```python
from build123d import *

# Parameters (mm, degrees)
SKETCH1_W                    = 152.4
SKETCH1_H                    = 50.8
BOSS_EXTRUDE2_DEPTH          = 152.4
SHELL1_T                     = -12.7
SKETCH2_R                    = 3.877794573
BOSS_EXTRUDE3_DEPTH          = 6
M2_5X0_45_TAPPED_HOLE3_D     = 2.05
M2_5X0_45_TAPPED_HOLE3_DEPTH = 4.99999
M2_5X0_45_TAPPED_HOLE3_TIP   = 0.615882135


with BuildPart() as part:
    # Sketch1 → Boss-Extrude2 (new body)
    with BuildSketch(Plane.XY):
        with Locations((65.122807232, 229.754701441)):
            Rectangle(SKETCH1_W, SKETCH1_H)
    extrude(amount=BOSS_EXTRUDE2_DEPTH)

    # Shell1
    shell1_openings = [part.faces().sort_by_distance(p)[0] for p in [
        (65.122807232, 255.154701441, 76.2),
    ]]
    offset(amount=SHELL1_T, openings=shell1_openings, kind=Kind.INTERSECTION)

    # Sketch2 → Boss-Extrude3 (add)
    with BuildSketch(Plane(origin=(0, 217.054701441, 0), x_dir=(1, 0, 0), z_dir=(0, 1, 0))):
        with Locations(Location((32.002807193, -55.2, 0), (0, 0, 270))):
            Circle(SKETCH2_R)
        with BuildLine():
            Line((99.91232539, -51.7), (96.573289151, -51.7))
            ThreePointArc((96.573289151, -51.7), (95.500792432, -57.942014839), (101.742807271, -56.869518119))
            Line((101.742807271, -56.869518119), (101.742807271, -53.530481881))
            ThreePointArc((101.742807271, -53.530481881), (100.984822109, -52.457985161), (99.91232539, -51.7))
        make_face()
        with BuildLine():
            ThreePointArc((33.672325312, -100.7), (34.744822031, -94.457985161), (28.502807193, -95.530481881))
            Line((28.502807193, -95.530481881), (28.502807193, -98.869518119))
            ThreePointArc((28.502807193, -98.869518119), (29.260792354, -99.942014839), (30.333289073, -100.7))
            Line((30.333289073, -100.7), (33.672325312, -100.7))
        make_face()
        with BuildLine():
            Line((101.742807271, -98.869518119), (101.742807271, -95.530481881))
            ThreePointArc((101.742807271, -95.530481881), (95.500792432, -94.457985161), (96.573289151, -100.7))
            Line((96.573289151, -100.7), (99.91232539, -100.7))
            ThreePointArc((99.91232539, -100.7), (100.984822109, -99.942014839), (101.742807271, -98.869518119))
        make_face()
    extrude(amount=BOSS_EXTRUDE3_DEPTH)

    # M2.5x0.45 Tapped Hole3
    with Locations(Plane(origin=(0, 223.054701441, 0), x_dir=(1, 0, 0), z_dir=(0, 1, 0))):
        with Locations((32.002807193, -55.2), (98.242807271, -55.2), (98.242807271, -97.2), (32.002807193, -97.2)):
            Hole(M2_5X0_45_TAPPED_HOLE3_D / 2, depth=M2_5X0_45_TAPPED_HOLE3_DEPTH)
            with Locations((0, 0, -(M2_5X0_45_TAPPED_HOLE3_DEPTH + M2_5X0_45_TAPPED_HOLE3_TIP / 2))):  # 118° drill point
                Cone(0, M2_5X0_45_TAPPED_HOLE3_D / 2, M2_5X0_45_TAPPED_HOLE3_TIP, mode=Mode.SUBTRACT)


solid = part.part
```
Source: CAD feature listing. Evaluate the final solid. Frame: model axes, mm. A direction names the side the tool comes from. Round coordinates to 2 decimals unless told otherwise and drop trailing zeros. Loops run counter-clockwise (first coordinate to the right, second up) from the corner with the lowest first, then second, coordinate; pieces in that order, holes last. Notation, with made-up numbers: M -30,50 L 21,50 A22 ccw 21,74 Z; hole C 23,34 d10. An arc over 180 degrees is marked long. Use a Markdown table: item, result. Add a question column.
1. Contact query for flat-ended pins moving along their axis: P1, Ø8, axis at x = 30.5, z = 95.5, coming from the +Y side; P2, Ø3, axis at x = 76.5, z = 115.5, coming from the +Y side. Output: stop coordinate, or through.
2. Section query A-A on y = 221. Give the number of separate pieces and of enclosed holes in the cut face, then the cut area to 3 significant figures.
3. Section query C-C on y = 242.5. Return the cut outline in (x, z), then the cut area to 3 significant figures.
4. Line query: line 1 (X direction, y = 220.1, z = 55.2); line 2 (X direction, y = 219, z = 55); line 3 (Z direction, x = 116.5, y = 249). Output: solid intervals per line, ascending.
5. Reachability of faces 1 (the flat face through (64, 204.355, 75)), 2 (the flat face through (97, 223.055, 55)) from +Z, -Z, +X, -X, +Y, -Y: full face, straight path, thin tool, end or side. Return the list, or none.
6. Mould query, pull axis X, two halves, no side actions, for faces 3 (the flat face through (141.323, 229, 75)), 4 (the flat face through (64, 230, 152.4)), 5 (the cylindrical face through (95.43, 220.01, 57.87)), 6 (the cylindrical face through (34.817, 220.013, 94.532)). Classes: pulls with the +X half, pulls with the -X half, needs draft (parallel to the pull), parting line crosses it, or undercut.
7. Section query D-D on z = 38.5. Return the cut outline in (x, y).
8. Section query B-B on x = 23. Return the cut outline in (y, z), then the cut area to 3 significant figures.
Reported:
| question | item | result |
|---|---|---|
| 1 | P1 | stops at y = 223.05 |
| 1 | P2 | stops at y = 217.05 |
| 2 | separate pieces | 5 |
| 2 | enclosed holes | 5 |
| 2 | area | 7,270 mm² |
| 3 | outline | M -11.08,0 L 141.32,0 L 141.32,152.4 L -11.08,152.4 Z; hole M 1.62,12.7 L 128.62,12.7 L 128.62,139.7 L 1.62,139.7 Z |
| 3 | area | 7,100 mm² |
| 4 | line 1 | x = -11.08 to 1.62, 28.13 to 30.98, 33.03 to 35.88, 94.37 to 97.22, 99.27 to 101.74, 128.62 to 141.32 |
| 4 | line 2 | x = -11.08 to 1.62, 28.13 to 31, 33.01 to 35.88, 94.37 to 97.24, 99.25 to 101.74, 128.62 to 141.32 |
| 4 | line 3 | z = 0 to 12.7, 139.7 to 152.4 |
| 5 | face 1 | +Z, -Z, +X, -X, -Y |
| 5 | face 2 | +Y |
| 6 | face 3 | pulls with the +X half |
| 6 | face 4 | needs draft |
| 6 | face 5 | undercut |
| 6 | face 6 | undercut |
| 7 | outline | M -11.08,204.35 L 141.32,204.35 L 141.32,255.15 L 128.62,255.15 L 128.62,217.05 L 1.62,217.05 L 1.62,255.15 L -11.08,255.15 Z |
| 8 | outline | M 204.35,0 L 255.15,0 L 255.15,12.7 L 217.05,12.7 L 217.05,139.7 L 255.15,139.7 L 255.15,152.4 L 204.35,152.4 Z |
| 8 | area | 2,900 mm² |
